```python
from build123d import *

# Parameters (mm, degrees)
SKETCH2_R               = 2.3495
SKETCH2_R_2             = 2.0955
BOSS_EXTRUDE1_DEPTH     = 2.54
SKETCH3_W               = 31.75
SKETCH3_H               = 44.323
BOSS_EXTRUDE2_DEPTH     = 2.54
SKETCH4_R               = 2.413
CUT_EXTRUDE1_DEPTH      = 238.743265275
SKETCH5_R               = 2.413
CUT_EXTRUDE2_DEPTH      = 238.743265275
SKETCH6_R               = 2.413
CUT_EXTRUDE3_DEPTH      = 238.743265275
SKETCH7_R               = 2.413
CUT_EXTRUDE4_DEPTH      = 238.743265275
SKETCH8_W               = 7.994763
SKETCH8_H               = 21.113506736
SKETCH8_W_2             = 21.493659396
SKETCH8_H_2             = 28.960940125
CUT_EXTRUDE5_DEPTH      = 238.743265275
CUT_EXTRUDE6_DEPTH      = 238.743265275
CUT_EXTRUDE6_DEPTH_BACK = 238.743265275


with BuildPart() as part:
    # Sketch2 → Boss-Extrude1 (new body)
    with BuildSketch(Plane(origin=(0, 0, 0), x_dir=(-1, 0, 0), z_dir=(0, 0, 1))):
        Polygon((-2.930050059, 168.708281075), (38.709428475, 168.708281075), (38.709428475, 189.536281075), (143.497061781, 189.536281075), (104.617436481, 110.859781075), (72.867436481, 110.859781075), (72.867436481, 66.536781075), (104.617436481, 66.536781075), (143.497061781, -12.139718925), (38.709428475, -12.139718925), (38.709428475, 8.688281075), (-2.930050059, 8.688281075), align=None)
        with Locations(Location((41.95655448, 160.961281075, 0), (0, 0, 180))):
            Circle(SKETCH2_R, mode=Mode.SUBTRACT)
        with Locations(Location((90.673911143, 180.011281075, 0), (0, 0, 180))):
            Circle(SKETCH2_R, mode=Mode.SUBTRACT)
        with Locations(Location((90.673911143, -2.614718925, 0), (0, 0, 180))):
            Circle(SKETCH2_R, mode=Mode.SUBTRACT)
        with Locations(Location((3.035061781, 117.209781075, 0), (0, 0, 180))):
            Circle(SKETCH2_R, mode=Mode.SUBTRACT)
        with Locations(Location((3.035061781, 60.186781075, 0), (0, 0, 180))):
            Circle(SKETCH2_R, mode=Mode.SUBTRACT)
        with Locations(Location((41.95655448, 16.435281075, 0), (0, 0, 180))):
            Circle(SKETCH2_R_2, mode=Mode.SUBTRACT)
    extrude(amount=BOSS_EXTRUDE1_DEPTH)

    # Sketch3 → Boss-Extrude2 (add)
    with BuildSketch(Plane.XY.offset(2.54)):
        with Locations((-88.742436481, -88.698281075)):
            Rectangle(SKETCH3_W, SKETCH3_H)
    extrude(amount=-BOSS_EXTRUDE2_DEPTH)

    # Sketch4 → Cut-Extrude1 (cut, through all)
    with BuildSketch(Plane.XY.offset(2.54)):
        with Locations((-94.457436481, -69.711781075)):
            Circle(SKETCH4_R)
        with Locations((-83.027436481, -69.711781075)):
            Circle(SKETCH4_R)
        with Locations((-28.311949941, -69.711781075)):
            Circle(SKETCH4_R)
        with Locations((-9.261949941, -69.711781075)):
            Circle(SKETCH4_R)
        with Locations(Location((-9.261949941, -107.684781075, 0), (0, 0, 180))):
            Circle(SKETCH4_R)
        with Locations(Location((-28.311949941, -107.684781075, 0), (0, 0, 180))):
            Circle(SKETCH4_R)
        with Locations(Location((-83.027436481, -107.684781075, 0), (0, 0, 180))):
            Circle(SKETCH4_R)
        with Locations(Location((-94.457436481, -107.684781075, 0), (0, 0, 180))):
            Circle(SKETCH4_R)
    extrude(amount=-CUT_EXTRUDE1_DEPTH, mode=Mode.SUBTRACT)

    # Sketch5 → Cut-Extrude2 (cut, through all)
    with BuildSketch(Plane.XY.offset(2.54)):
        with Locations((-31.738991634, -58.273080522)):
            Circle(SKETCH5_R)
    extrude(amount=-CUT_EXTRUDE2_DEPTH, mode=Mode.SUBTRACT)

    # Sketch6 → Cut-Extrude3 (cut, through all)
    with BuildSketch(Plane.XY.offset(2.54)):
        with Locations((-32.511395831, -23.991781075)):
            Circle(SKETCH6_R)
    extrude(amount=-CUT_EXTRUDE3_DEPTH, mode=Mode.SUBTRACT)

    # Sketch7 → Cut-Extrude4 (cut, through all)
    with BuildSketch(Plane.XY.offset(2.54)):
        with Locations((-32.140467993, -155.071444629)):
            Circle(SKETCH7_R)
        with Locations((-32.140467993, -120.781444629)):
            Circle(SKETCH7_R)
    extrude(amount=-CUT_EXTRUDE4_DEPTH, mode=Mode.SUBTRACT)

    # Sketch8 → Cut-Extrude5 (cut, through all)
    with BuildSketch(Plane.XY.offset(2.54)):
        with Locations((-36.236046975, 1.868472293)):
            Rectangle(SKETCH8_W, SKETCH8_H)
        with Locations((-29.486598777, -183.188751137)):
            Rectangle(SKETCH8_W_2, SKETCH8_H_2)
    extrude(amount=-CUT_EXTRUDE5_DEPTH, mode=Mode.SUBTRACT)

    # Sketch9 → Cut-Extrude6 (cut, two sides: drawn at the far end of the back side and taken through both)
    with BuildSketch(Plane.XY.offset(2.54).offset(-CUT_EXTRUDE6_DEPTH_BACK)):
        Polygon((-104.617436481, -66.536781075), (-104.617436481, 15.636566552), (-183.179161499, 15.636566552), (-188.262141255, -199.721259961), (-104.617436481, -202.664037714), align=None)
    extrude(amount=CUT_EXTRUDE6_DEPTH + CUT_EXTRUDE6_DEPTH_BACK, mode=Mode.SUBTRACT)


solid = part.part
```
Could you check a few things on this model? Use its own coordinates, in mm. Round coordinates to 2 decimals unless told otherwise and drop trailing zeros.
Q1. Thinking about a two-plate mould opening in X: for faces 1 (the flat face through (-52, -87, 2.54)), 2 (the cylindrical face through (-8.148, -71.853, 1.288)), which applies, pulls with the +X half, pulls with the -X half, needs draft (parallel to the pull), parting line crosses it, or undercut?
Q2. I want a section at A-A (z = 0.7). Give the number of separate pieces and of enclosed holes in the cut face, and give its area (3 significant figures).
Q3. Please list where these lines run through material, in increasing order: L1, parallel to Y at x = -3.5, z = 1.6; L2, parallel to Y at x = -42, z = 0.6; L3, parallel to Y at x = -33, z = 1.8.
Q4. For P1, Ø3, axis at x = -90.67, y = 2.61, coming from the +Z side; P2, Ø0.8, axis at x = -8, z = 1.5, coming from the -Y side, each with a flat end and sliding along its axis, tell me the tip position at first contact or that it passes through.
Answer below:
1. face 1: needs draft
1. face 2: undercut
2. separate pieces: 1
2. enclosed holes: 18
2. area: 19,600 mm2
3. L1: y = -168.71 to -119.51, -114.91 to -62.49, -57.88 to -8.69
3. L2: y = -189.54 to -163.31, -158.61 to -18.53, -14.34 to 12.14
3. L3: y = -168.71 to -157.33, -152.82 to -123.04, -118.53 to -60.33, -56.22 to -26.35, -21.63 to -8.69
4. P1: passes through
4. P2: stops at y = -168.71
